Can you work these out from the drawing? Everything is in mm from the part's minimum corner. A direction names the side the tool comes from. Round coordinates to 2 decimals unless told otherwise and drop trailing zeros. Loops run counter-clockwise (first coordinate to the right, second up) from the corner with the lowest first, then second, coordinate; pieces in that order, holes last. Notation, with made-up numbers: M 69.5,18.5 L 123.5,18.5 A11 cw 123.5,35.5 Z; hole C 1.5,52.25 d9. An arc over 180 degrees is marked long. Use a Markdown table: item, result.
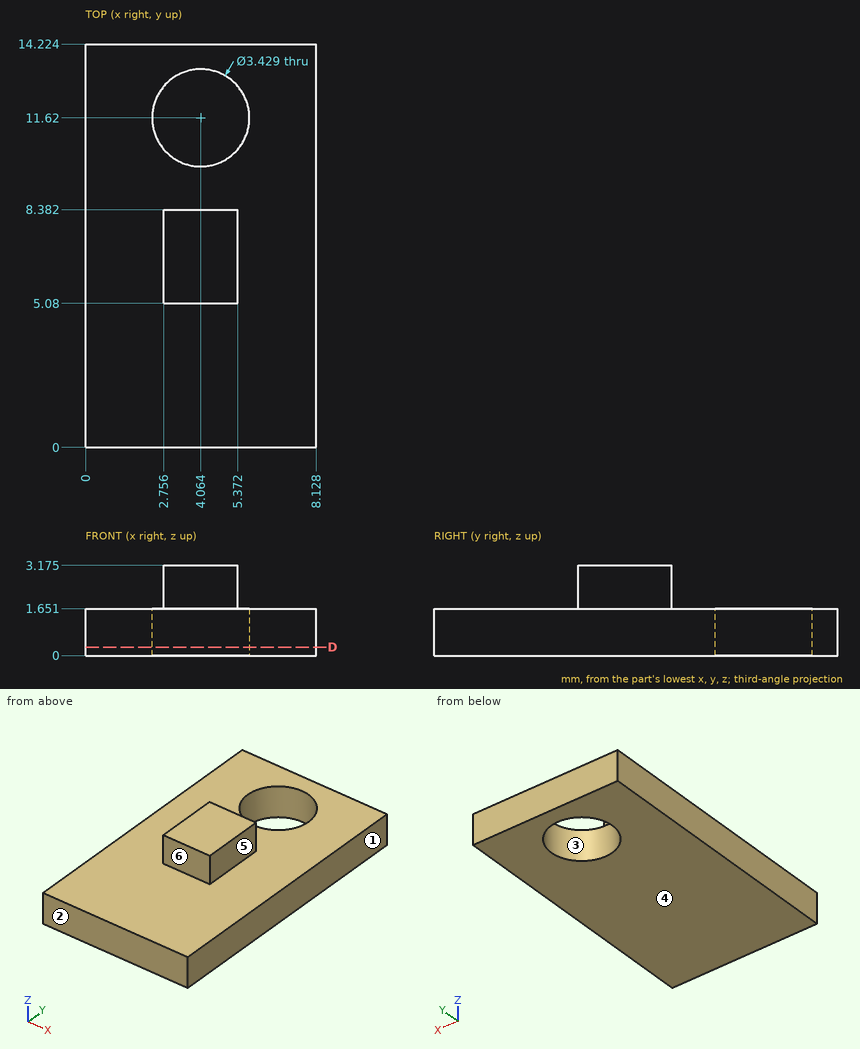
1. For pin 1 Ø0.5 at (y, z) = (6.5, 2.5) entering from -X; pin 2 Ø0.5 at (x, z) = (3.5, 2.5) entering from -Y; pin 3 Ø3 at (x, y) = (7, 3) entering from +Z; pin 4 Ø4 at (x, y) = (4.06, 11.62) entering from -Z, each with a flat end and sliding along its axis, tell me the tip position at first contact or that it passes through.
Answer sheet:
| item | result |
|---|---|
| pin 1 | x = 2.76 |
| pin 2 | y = 5.08 |
| pin 3 | z = 1.65 |
| pin 4 | z = 0 |
2. Which directions (+Z, -Z, +X, -X, +Y, -Y) give clear straight access to the entire face, cutting with the end or side of a thin tool? Please do the marked faces 4, 5 and 6.
Answer sheet:
| item | result |
|---|---|
| face 4 | -Z, +X, -X, +Y, -Y |
| face 5 | +Z, +X, +Y, -Y |
| face 6 | +Z, +X, -X, -Y |
3. I need wall thicknesses on probe 1 along Z at (x, y) = (6, 9.5); probe 2 along Y at (x, z) = (4, 1.8); probe 3 along X at (y, z) = (7.75, 2.5) (1 decimal). Which ranges of each line are inside material? Lowest first, please. Write a range as from..to.
Answer sheet:
| item | result |
|---|---|
| probe 1 | 0..1.65 |
| probe 2 | 5.08..8.38 |
| probe 3 | 2.8..5.4 |
4. Imagine slicing it at D-D, the plane z = 0.3. Write out the boundary of the cut face in (x, y) (1 decimal).
Answer sheet:
| item | result |
|---|---|
| outline | M 0,0 L 8.1,0 L 8.1,14.2 L 0,14.2 Z; hole C 4.1,11.6 d3.4 |
5. We'd pull the mould along Y, two halves only. Please class the marked faces 1, 2 and 3: +Y half, -Y half, draft (parallel to the pull), parting line (faces both ways), or undercut.
Answer sheet:
| item | result |
|---|---|
| face 1 | draft |
| face 2 | -Y half |
| face 3 | undercut |
